from build123d import *

# Parameters (mm, degrees)
P_IDAT_VYSUNUT_M1_DEPTH  = 5.555
P_IDAT_VYSUNUT_M2_DEPTH  = 4
SKICA3_R                 = 2.03883748
SKICA3_R_2               = 1.24519559
P_IDAT_VYSUNUT_M3_DEPTH  = 3
SKICA5_R                 = 1.190602913
SKICA5_R_2               = 1.19060243
ODEBRAT_VYSUNUT_M1_DEPTH = 23
SKICA7_W                 = 1
SKICA7_H                 = 4
P_IDAT_VYSUNUT_M4_DEPTH  = 1


# Read off the part's stored shape, not the designer's step: Přidat vysunutím2
with BuildPart() as part:
    # Skica1 → Přidat vysunutím1 (new, symmetric)
    with BuildSketch(Plane(origin=(0, 0, 0), x_dir=(1, 0, 0), z_dir=(0, 1, 0))):
        Polygon((11.32935, -15.875), (16.09185, -15.875), (16.09185, -18.25625), (11.32935, -18.25625), (11.32935, -22.225), (-10.89565, -22.225), (-10.89565, -18.25625), (-15.65815, -18.25625), (-15.65815, -15.875), (-10.89565, -15.875), (-10.89565, 0), (11.32935, 0), align=None)
    extrude(amount=P_IDAT_VYSUNUT_M1_DEPTH, both=True)

    # Přidat vysunutím2 outline → Přidat vysunutím2 (add)
    with BuildSketch(Plane.XY.offset(22.225)):
        with BuildLine():
            Line((-10.89565, 0.263816958), (-10.89565, -0.263816958))
            ThreePointArc((-10.89565, -0.263816958), (-6.494080203, -5.390484118), (-0.444197365, -2.381256561))
            Line((-0.444197365, -2.381256561), (1.010536018, -2.381256561))
            ThreePointArc((1.010536018, -2.381256561), (3.391829299, 2.729e-06), (1.010604, 2.38133))
            Line((1.010604, 2.38133), (-0.444232639, 2.38133))
            ThreePointArc((-0.444232639, 2.38133), (-6.494120128, 5.390476029), (-10.89565, 0.263816958))
        make_face()
    extrude(amount=P_IDAT_VYSUNUT_M2_DEPTH)

    # Skica3 → Přidat vysunutím3 (add)
    with BuildSketch(Plane.XY.offset(26.225)):
        with Locations((-5.401980861, 0)):
            Circle(SKICA3_R)
        with Locations((-5.401980861, 0)):
            Circle(SKICA3_R_2, mode=Mode.SUBTRACT)
    extrude(amount=P_IDAT_VYSUNUT_M3_DEPTH)

    # Skica5 → Odebrat vysunutím1 (cut)
    with BuildSketch(Plane.XY.offset(18.25625)):
        with Locations((-13.276937552, 5.8558e-05)):
            Circle(SKICA5_R)
        with Locations((13.71053658, 6.1415e-05)):
            Circle(SKICA5_R_2)
    extrude(amount=-ODEBRAT_VYSUNUT_M1_DEPTH, mode=Mode.SUBTRACT)

    # Skica7 → Přidat vysunutím4 (add)
    with BuildSketch(Plane(origin=(-10.89565, 0, 10.89565), x_dir=(0, 0, -1), z_dir=(1, 0, 0))):
        with Locations((7.39565, 0)):
            Rectangle(SKICA7_W, SKICA7_H)
    extrude(amount=-P_IDAT_VYSUNUT_M4_DEPTH)


solid = part.part
Could you check a few things on this model? Use its own coordinates, in mm. A direction names the side the tool comes from. Give positions to 0.01 mm unless a question says otherwise; leave off trailing zeros. Order: outer loops, then holes, each group sorted by start corner. A loop starts at its lowest first (then second) coordinate and runs counter-clockwise, first axis right, second up. Notation, with made-up numbers: (-36, 56) - (12, 56) arc R11 ccw to (12, 60) - close; hole circle Ø4 at (55.25, -39.5). An arc over 180 degrees is marked (long way). One line per question, with ' | ' between items. Start each with the question number.
Item 1: For faces 1 (the cylindrical face through (3.39, -0.05, 24.2)), 2 (the flat face through (-10.896, 0, 21)), 3 (the flat face through (11.329, 0, 8)), which set-ups out of +Z, -Z, +X, -X, +Y, -Y let a thin tool reach every point of the face, with its end or its side?
Item 2: I need wall thicknesses on probe 1 along Z at (x, y) = (5, 3.25) (3 decimals); probe 2 along Z at (x, y) = (11.5, -3.75) (3 decimals); probe 3 along X at (y, z) = (-2.5, 21.25). Which ranges of each line are inside material? Lowest first, please. Write a range as [from, to].
Item 3: I'm going to push flat-ended pins straight in: pin 1 Ø1.1 at (x, z) = (-11.5, 3.5) entering from -Y; pin 2 Ø4 at (x, y) = (-13.5, 1.5) entering from +Z; pin 3 Ø2.5 at (x, y) = (12.5, 0.5) entering from +Z (3 decimals); pin 4 Ø2 at (x, y) = (-13.28, 0) entering from +Z. Where does each tip first touch, or does it pass through?
Item 4: I want a section at C-C on z = 17.5. Write out the boundary of the cut face in (x, y) (3 decimals).
Item 5: I want a section at B-B on y = 3. Write out the boundary of the cut face in (x, z) (3 decimals), then the cut area to 3 significant figures.
Item 6: I want a section at A-A on z = 24.25. Write out the boundary of the cut face in (x, y), then the cut area to 3 significant figures.
Item 7: Thinking about a two-plate mould opening in Y: for faces 4 (the flat face through (-5, 0, 26.225)), 5 (the flat face through (11.329, 0, 20)), 6 (the flat face through (0, -2.381, 24)), which applies, pulls with the +Y half, pulls with the -Y half, needs draft (parallel to the pull), parting line crosses it, or undercut?
Item 8: I want a section at D-D on x = 7. Write out the boundary of the cut face in (y, z) (3 decimals).
Verdict:
1) face 1: +Z, +X | face 2: +Z, -X, +Y, -Y | face 3: -Z, +X, +Y, -Y
2) probe 1: [0, 22.225] | probe 2: [15.875, 18.256] | probe 3: [-10.9, 11.33]
3) pin 1: y = -2 | pin 2: z = 18.26 | pin 3: z = 22.225 | pin 4: through
4) outline: (-15.658, -5.555) - (16.092, -5.555) - (16.092, 5.555) - (-15.658, 5.555) - close; hole circle Ø2.381 at (-13.277, 0); hole circle Ø2.381 at (13.711, 0)
5) outline: (-15.658, 15.875) - (-10.896, 15.875) - (-10.896, 0) - (11.329, 0) - (11.329, 15.875) - (16.092, 15.875) - (16.092, 18.256) - (11.329, 18.256) - (11.329, 22.225) - (-0.792, 22.225) - (-0.792, 26.225) - (-10.012, 26.225) - (-10.012, 22.225) - (-10.896, 22.225) - (-10.896, 18.256) - (-15.658, 18.256) - close | area: 554 mm^2
6) outline: (-10.9, -0.26) arc R5.5 ccw to (-0.44, -2.38) - (1.01, -2.38) arc R2.38 ccw to (1.01, 2.38) - (-0.44, 2.38) arc R5.5 ccw to (-10.9, 0.26) - close | area: 109 mm^2
7) face 4: undercut | face 5: needs draft | face 6: pulls with the -Y half
8) outline: (-5.555, 0) - (5.555, 0) - (5.555, 22.225) - (-5.555, 22.225) - close
